```python
from build123d import *

# Parameters (mm, degrees)
BOSS_EXTRUDE1_DEPTH = 5


with BuildPart() as part:
    # Sketch1 → Boss-Extrude1 (new body)
    with BuildSketch(Plane(origin=(0, 0, 0), x_dir=(1, 0, 0), z_dir=(0, 1, 0))):
        with BuildLine():
            Line((8.75, -2.5), (14.25, -2.5))
            Line((14.25, -2.5), (14.25, -72.5))
            ThreePointArc((14.25, -72.5), (12.785533906, -76.035533906), (9.25, -77.5))
            Line((9.25, -77.5), (-9.25, -77.5))
            ThreePointArc((-9.25, -77.5), (-12.785533906, -76.035533906), (-14.25, -72.5))
            Line((-14.25, -72.5), (-14.25, -2.5))
            Line((-14.25, -2.5), (-8.75, -2.5))
            Line((-8.75, -2.5), (-8.75, 2.5))
            Line((-8.75, 2.5), (8.75, 2.5))
            Line((8.75, 2.5), (8.75, -2.5))
        make_face()
    extrude(amount=BOSS_EXTRUDE1_DEPTH)


solid = part.part
```
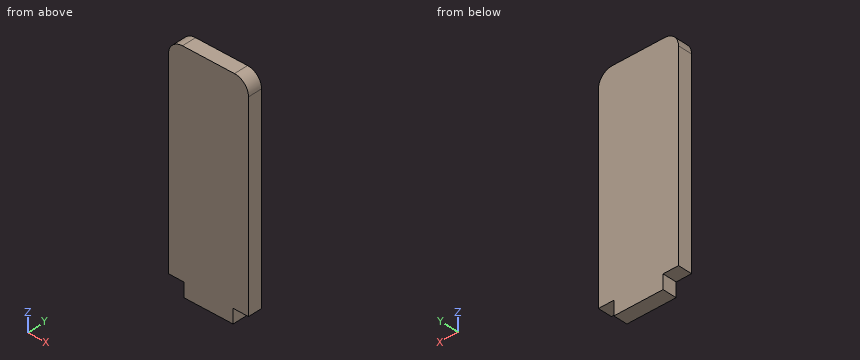
The model under review builds one solid part; all positions refer to its coordinate system, in mm. Round coordinates to 2 decimals unless told otherwise and drop trailing zeros. Write each loop counter-clockwise with the first axis right and the second up, starting at its lowest first coordinate (ties: lowest second). Pieces come first, ordered by that corner, then holes. Notation, with made-up numbers: (18.25, 65) -> (28.25, 65) arc R24 ccw to (28.25, 83) -> close; hole circle Ø7 at (60.5, 35). An arc over 180 degrees is marked (long way). Use CSV: the item, a comma, the result in double quotes.
Q1. To check wall thickness, follow probe 1 along Z at (x, y) = (13, 3.7); probe 2 along Z at (x, y) = (10.5, 3.25). State the ranges of each line that lie inside material, in increasing order. Write a range as [from, to].
Checks:
probe 1,"[2.5, 75.81]"
probe 2,"[2.5, 77.34]"
Q2. Consider section A-A (y = 3.5). Give the boundary of the cut face in (x, z).
Checks:
outline,"(-14.25, 2.5) -> (-8.75, 2.5) -> (-8.75, -2.5) -> (8.75, -2.5) -> (8.75, 2.5) -> (14.25, 2.5) -> (14.25, 72.5) arc R5 ccw to (9.25, 77.5) -> (-9.25, 77.5) arc R5 ccw to (-14.25, 72.5) -> close"
Q3. For pin 1 Ø1.5 at (x, y) = (-11, 1.5) entering from -Z; pin 2 Ø2.5 at (y, z) = (2, 0) entering from -X, all flat-tipped, find the tip position at first contact; note any pin that passes through.
Checks:
pin 1,"z = 2.5"
pin 2,"x = -8.75"
